Autodesk Inventor part; units mm, degrees
ref_plane "YZ Plane" through (0, 0, 0) normal (1, 0, 0) x (0, 1, 0)
ref_plane "XZ Plane" through (0, 0, 0) normal (0, 1, 0) x (-1, 0, 0)
ref_plane "XY Plane" through (0, 0, 0) normal (0, 0, 1) x (1, 0, 0)
ref_plane "РабПлоскость1" through (-194.4569, -1.6478, -98.8355) normal (0, 0, 1) x (0, -1, 0)
sketch "Эскиз1" plane through (-194.4569, -1.6478, -98.8355) normal (0, 0, 1) x (0, -1, 0)
  circle A0 centre (5, 145) radius 1.5
  circle A1 centre (5, 119) radius 1.5
  circle A2 centre (18, 132) radius 7
  circle A3 centre (31, 119) radius 1.5
  circle A4 centre (31, 145) radius 1.5
  line L0 (18.8381, 124.6132) -> (31, 119)
  line L1 (17.1619, 124.6132) -> (5, 119)
  line L2 (5, 119) -> (10.6132, 131.1619)
  line L3 (5, 145) -> (10.6132, 132.8381)
  line L4 (17.1619, 139.3868) -> (5, 145)
  line L5 (18.8381, 139.3868) -> (31, 145)
  line L6 (31, 145) -> (25.3868, 132.8381)
  line L7 (25.3868, 131.1619) -> (31, 119)
  circle A5 centre (5, 119) radius 5.275
  circle A6 centre (5, 145) radius 5.275
  circle A7 centre (31, 145) radius 5.275
  circle A8 centre (31, 119) radius 5.275
  arc A9 (18.8381, 124.6132) -> (17.1619, 124.6132) centre (18, 122.7973) ccw
  arc A10 (25.3868, 132.8381) -> (25.3868, 131.1619) centre (27.2027, 132) ccw
  arc A11 (17.1619, 139.3868) -> (18.8381, 139.3868) centre (18, 141.2027) ccw
  arc A12 (10.6132, 131.1619) -> (10.6132, 132.8381) centre (8.7973, 132) ccw
  circle A13 centre (18, 132) radius 2.75
  point P0 (-1.6478, 194.4569)
  point P1 (18, 125)
  point P2 (11, 132)
  point P3 (18, 139)
  point P4 (25, 132)
  point P5 (9.7895, 121.2105)
  point P6 (26.2105, 121.2105)
  point P7 (28.7895, 123.7895)
  point P8 (28.7895, 140.2105)
  point P9 (26.2105, 142.7895)
  point P10 (9.7895, 142.7895)
  point P11 (7.2105, 140.2105)
  point P12 (7.2105, 123.7895)
  point P13 (6.3619, 119.6286)
  point P14 (5.6286, 120.3619)
  point P15 (5.6286, 143.6381)
  point P16 (6.3619, 144.3714)
  point P17 (29.6381, 144.3714)
  point P18 (30.3714, 143.6381)
  point P19 (30.3714, 120.3619)
  point P20 (29.6381, 119.6286)
  dimension "d0" = 2
  dimension "d1" = 5.5
extrude "Выдавливание1" add sketch "Эскиз1" along normal blind 2 contours A0 L3 A6 L4 | A0 L4 A6 L3 | A6 L4 A11 L5 A7 L6 A10 L7 A8 L0 A9 L1 A5 L2 A12 L3 | A5 L1 A1 L2 | L2 A1 L1 A5 | A7 L6 A4 L5 | L5 A4 L6 A7 | A8 L7 A3 L0 | L0 A3 L7 A8 | A2
properties part number "крепеж подшипника"
Verification items for the finished model (mm, model axes). Coordinates: 2 decimals unless noted, no trailing zeros. Order: outer loops, then holes, each group sorted by start corner. A loop starts at its lowest first (then second) coordinate and runs counter-clockwise, first axis right, second up. Notation, with made-up numbers: (69, 61) -> (101, 61) arc R34 cw to (101, 95) -> close; hole circle Ø5 at (-13, 9). An arc over 180 degrees is marked (long way). Answer as CSV lines item,"result". Start each with the question number.
1) Cross-section at B-B, the plane y = -28.5. Record the boundary of the cut face in (x, z).
2) Gauge pin test, flat ends, axial feed: pin 1 Ø6 at (x, y) = (-63, -6.5) entering from +Z; pin 2 Ø1 at (x, z) = (-70.5, -97.5) entering from -Y; pin 3 Ø5 at (x, y) = (-49.46, -6.65) entering from +Z; pin 4 Ø1 at (x, z) = (-68.5, -97) entering from +Y. Record the tip position at first contact, or that the pin passes through.
3) Material ranges on L1, parallel to Y at x = -49.5, z = -98.1; L2, parallel to X at y = -7, z = -97.1; L3, parallel to X at y = -19.5, z = -97.05, recorded low to high. Write a range as [from, to].
4) Cross-section at D-D, the plane x = -59. Record the boundary of the cut face in (y, z).
5) Cross-section at A-A, the plane x = -64.5. Record the boundary of the cut face in (y, z), then the cut area to 3 significant figures.
6) Cross-section at C-C, the plane z = -97.55. Give the number of separate pieces and of enclosed holes in the cut face, then the cut area to 3 significant figures.
7) Release check for a two-part mould opening along Y. For faces 1 (the face through (-62.445, -12.445, -97.849)), 2 (the face through (-62.47, -26.85, -97.85)), 3 (the face through (-69.66, -19.64, -97.85)) record: released by +Y, released by -Y, zero draft, split by the parting line, or undercut.
Conclusion:
1,outline,"(-78.72, -98.84) -> (-66.47, -98.84) -> (-66.47, -96.84) -> (-78.72, -96.84) -> close; (-58.44, -98.84) -> (-46.2, -98.84) -> (-46.2, -96.84) -> (-58.44, -96.84) -> close"
2,pin 1,"passes through"
2,pin 2,"stops at y = -35.47"
2,pin 3,"stops at z = -96.84"
2,pin 4,"stops at y = -9.63"
3,L1,"y = [-37.92, -34.15], [-31.15, -27.37], [-11.92, -8.15], [-5.15, -1.37]"
3,L2,"x = [-80.72, -76.91], [-74, -70.19], [-54.72, -50.91], [-48, -44.19]"
3,L3,"x = [-69.67, -65.2], [-59.71, -55.25]"
4,outline,"(-28.24, -98.84) -> (-11.05, -98.84) -> (-11.05, -96.84) -> (-28.24, -96.84) -> close"
5,outline,"(-27.59, -98.84) -> (-21.49, -98.84) -> (-21.49, -96.84) -> (-27.59, -96.84) -> close; (-17.81, -98.84) -> (-11.7, -98.84) -> (-11.7, -96.84) -> (-17.81, -96.84) -> close"
5,area,"24.4 mm²"
6,separate pieces,"1"
6,enclosed holes,"5"
6,area,"623 mm²"
7,face 1,"released by +Y"
7,face 2,"released by -Y"
7,face 3,"undercut"
